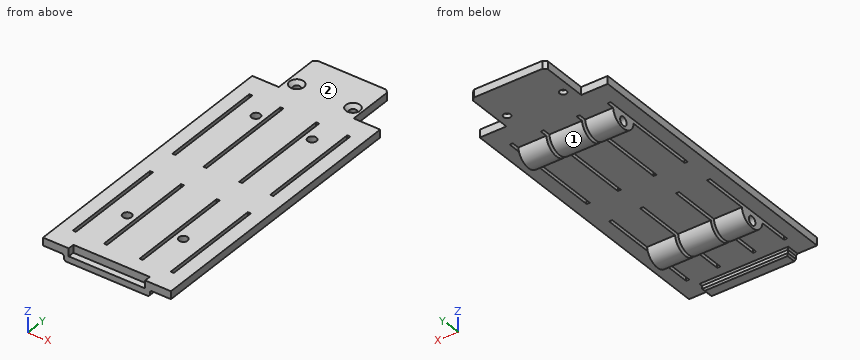
```python
from build123d import *

# Parameters (mm, degrees)
BOSS_EXTRU_1_DEPTH              = 2.5
BOSS_EXTRU_2_DEPTH              = 30.59
ESQUISSE5_W                     = 2
ESQUISSE5_H                     = 67
ENL_V_MAT_EXTRU_1_DEPTH         = 130.359962894
ESQUISSE14_W                    = 49
ESQUISSE14_H                    = 4
ENL_V_MAT_EXTRU_5_DEPTH         = 129.953479984
R_P_TITION_LIN_AIRE2_COUNT      = 2
R_P_TITION_LIN_AIRE2_PITCH      = 19.921
ESQUISSE17_R                    = 2.25
ENL_V_MAT_EXTRU_7_DEPTH         = 10
ESQUISSE15_W                    = 55
ESQUISSE15_H                    = 7
BOSS_EXTRU_4_DEPTH              = 4
CHANFREIN3_SIZE                 = 1
CHANFREIN4_SIZE                 = 2
ESQUISSE19_R                    = 2.8
ENL_V_MAT_EXTRU_9_DEPTH         = 8
CHANFREIN5_SIZE                 = 2.3
SYM_TRIE9_COPY_1_SKETCH_W       = 2
SYM_TRIE9_COPY_1_SKETCH_H       = 67
SYM_TRIE9_COPY_1_DEPTH          = 130.359962894
ESQUISSE20_R                    = 2.8
ENL_V_MAT_EXTRU_10_DEPTH        = 10
R_P_TITION_LIN_AIRE3_COUNT      = 2
R_P_TITION_LIN_AIRE3_PITCH      = 36
R_P_TITION_LIN_AIRE3_COUNT_DIR2 = 2
R_P_TITION_LIN_AIRE3_PITCH_DIR2 = 112


with BuildPart() as part:
    # Esquisse1 → Boss.-Extru.1 (new, symmetric)
    with BuildSketch(Plane.XY):
        Polygon((-41, -91), (-15.008, -91), (41, -91), (41, 91), (24, 91), (24, 122), (-24, 122), (-24, 91), (-41, 91), align=None)
    extrude(amount=BOSS_EXTRU_1_DEPTH, both=True)

    # Esquisse6 → Boss.-Extru.2 (add, symmetric)
    with BuildSketch(Plane(origin=(0, 0, 0), x_dir=(0, 0, -1), z_dir=(1, 0, 0))):
        with BuildLine():
            Line((2.5, -57.94427191), (2.5, -40.05572809))
            ThreePointArc((2.5, -40.05572809), (10.5, -49), (2.5, -57.94427191))
        make_face()
        with BuildLine():
            Line((2.5, 54.05572809), (2.5, 71.94427191))
            ThreePointArc((2.5, 71.94427191), (10.5, 63), (2.5, 54.05572809))
        make_face()
    extrude(amount=BOSS_EXTRU_2_DEPTH, both=True)

    # Esquisse5 → Enlèv. mat.-Extru.1 (cut, symmetric)
    with BuildSketch(Plane.XY.offset(2.5)):
        with Locations((31.3815, -43.25)):
            Rectangle(ESQUISSE5_W, ESQUISSE5_H)
        with Locations((31.3815, 43.25)):
            Rectangle(ESQUISSE5_W, ESQUISSE5_H)
    enl_v_mat_extru_1 = extrude(amount=ENL_V_MAT_EXTRU_1_DEPTH, both=True, mode=Mode.SUBTRACT)

    # Esquisse14 → Enlèv. mat.-Extru.5 (cut, through all)
    with BuildSketch(Plane(origin=(0, 0, -2.5), x_dir=(-1, 0, 0), z_dir=(0, 0, -1))):
        with Locations((0, -89)):
            Rectangle(ESQUISSE14_W, ESQUISSE14_H)
    extrude(amount=-ENL_V_MAT_EXTRU_5_DEPTH, mode=Mode.SUBTRACT)

    # Répétition linéaire2: Enlèv. mat.-Extru.1 ×2
    with Locations(*[(-i * R_P_TITION_LIN_AIRE2_PITCH, 0, 0) for i in range(1, R_P_TITION_LIN_AIRE2_COUNT)]):
        add(enl_v_mat_extru_1, mode=Mode.SUBTRACT)

    # Esquisse17 → Enlèv. mat.-Extru.7 (cut)
    with BuildSketch(Plane.XY.offset(2.5)):
        with Locations((18, 98.55)):
            Circle(ESQUISSE17_R)
        with Locations((-18, 98.55)):
            Circle(ESQUISSE17_R)
    extrude(amount=-ENL_V_MAT_EXTRU_7_DEPTH, mode=Mode.SUBTRACT)

    # Esquisse15 → Boss.-Extru.4 (add)
    with BuildSketch(Plane(origin=(0, 0, -2.5), x_dir=(-1, 0, 0), z_dir=(0, 0, -1))):
        with Locations((0, -87.5)):
            Rectangle(ESQUISSE15_W, ESQUISSE15_H)
    extrude(amount=BOSS_EXTRU_4_DEPTH)

    # Chanfrein3
    chanfrein3_edges = [part.edges().sort_by_distance(p)[0] for p in [
        (27.5, -87.5, -2.5),
        (-27.5, -87.5, -2.5),
        (0, -84, -2.5),
        (27.5, -87.5, -6.5),
        (-27.5, -87.5, -6.5),
        (0, -84, -6.5),
    ]]
    chamfer(chanfrein3_edges, length=CHANFREIN3_SIZE)

    # Chanfrein4
    chanfrein4_edges = [part.edges().sort_by_distance(p)[0] for p in [
        (-24, 122, 0),
        (24, 122, 0),
    ]]
    chamfer(chanfrein4_edges, length=CHANFREIN4_SIZE)

    # Esquisse19 → Enlèv. mat.-Extru.9 (cut)
    with BuildSketch(Plane(origin=(30.3815, 0, 0), x_dir=(0, 0, -1), z_dir=(1, 0, 0))):
        with Locations(Location((6, 63, 0), (0, 0, 90))):
            Circle(ESQUISSE19_R)
        with Locations(Location((6, -49, 0), (0, 0, 90))):
            Circle(ESQUISSE19_R)
    enl_v_mat_extru_9 = extrude(amount=-ENL_V_MAT_EXTRU_9_DEPTH, mode=Mode.SUBTRACT)

    # Symétrie8: Enlèv. mat.-Extru.9 across plane
    add(enl_v_mat_extru_9.mirror(Plane(origin=(0, 0, 0), x_dir=(0, 0, 1), z_dir=(1, 0, 0))), mode=Mode.SUBTRACT)

    # Chanfrein5
    chanfrein5_edges = [part.edges().sort_by_distance(p)[0] for p in [
        (15.75, 98.55, 2.5),
        (-20.25, 98.55, 2.5),
    ]]
    chamfer(chanfrein5_edges, length=CHANFREIN5_SIZE)

    # Symétrie9: Enlèv. mat.-Extru.1 across plane
    add(enl_v_mat_extru_1.mirror(Plane(origin=(0, 0, 0), x_dir=(0, 0, 1), z_dir=(1, 0, 0))), mode=Mode.SUBTRACT)

    # Symétrie9 copy 1 sketch → Symétrie9 copy 1 (cut, symmetric)
    with BuildSketch(Plane(origin=(19.921, 0, 2.5), x_dir=(-1, 0, 0), z_dir=(0, 0, 1))):
        with Locations((31.3815, 43.25)):
            Rectangle(SYM_TRIE9_COPY_1_SKETCH_W, SYM_TRIE9_COPY_1_SKETCH_H)
        with Locations((31.3815, -43.25)):
            Rectangle(SYM_TRIE9_COPY_1_SKETCH_W, SYM_TRIE9_COPY_1_SKETCH_H)
    extrude(amount=SYM_TRIE9_COPY_1_DEPTH, both=True, mode=Mode.SUBTRACT)

    # Esquisse20 → Enlèv. mat.-Extru.10 (cut)
    with BuildSketch(Plane.XY.offset(2.5)):
        with Locations((-18, -49)):
            Circle(ESQUISSE20_R)
    enl_v_mat_extru_10 = extrude(amount=-ENL_V_MAT_EXTRU_10_DEPTH, mode=Mode.SUBTRACT)

    # Répétition linéaire3: Enl_v. mat.-Extru.10 2 × 2
    with Locations(*[(i * R_P_TITION_LIN_AIRE3_PITCH, j * R_P_TITION_LIN_AIRE3_PITCH_DIR2, 0) for i in range(R_P_TITION_LIN_AIRE3_COUNT) for j in range(R_P_TITION_LIN_AIRE3_COUNT_DIR2) if (i, j) != (0, 0)]):
        add(enl_v_mat_extru_10, mode=Mode.SUBTRACT)


solid = part.part
```
Source: CAD feature listing. Evaluate the final solid. Frame: model axes, mm. Face numbers are marked on the shaded views. Give positions to 0.01 mm unless a question says otherwise; leave off trailing zeros. Order: outer loops, then holes, each group sorted by start corner. A loop starts at its lowest first (then second) coordinate and runs counter-clockwise, first axis right, second up.
(1) Section query C-C (x = 1). Return the cut outline in (y, z).
(2) Contact query for flat-ended pins moving along their axis: P1, Ø3.5, axis at x = 18, y = 63, coming from the +Z side; P2, Ø5.5, axis at y = 110, z = 0, coming from the +X side; P3, Ø2, axis at y = -45, z = -5.5, coming from the -X side; P4, Ø6.5, axis at y = 44, z = -6.5, coming from the +X side. Output: stop coordinate, or through.
(3) Section query B-B (y = 98.55). Return the cut outline in (x, z).
(4) Material intervals for line 1 along Y through (x, z) = (-18, -1.4); line 2 along X through (y, z) = (72, -1.5); line 3 along Y through (x, z) = (-18, -5.5), sorted ascending.
(5) Section query D-D (y = 63). State how many separate pieces and enclosed holes the cut face has, plus the area to 3 significant figures.
(6) Pull-direction query (Y, two-part tool) for the marked faces 1 and 2; classes: +Y half, -Y half, draft (parallel to the pull), parting line (faces both ways), or undercut.
(7) Section query A-A (x = 18). Return the cut outline in (y, z).
Outcome:
1. outline: (-91, -6.5) - (-85, -6.5) - (-84, -5.5) - (-84, -3.5) - (-83, -2.5) - (-57.94, -2.5) arc R9 ccw to (-40.06, -2.5) - (54.06, -2.5) arc R9 ccw to (71.94, -2.5) - (122, -2.5) - (122, 2.5) - (-87, 2.5) - (-87, -2.5) - (-91, -2.5) - close
2. P1: stops at z = -7.5
2. P2: stops at x = 24
2. P3: stops at x = -30.38
2. P4: passes through
3. outline: (-24, -2.5) - (-20.25, -2.5) - (-20.25, 0.2) - (-22.55, 2.5) - (-24, 2.5) - close; (-15.75, -2.5) - (15.75, -2.5) - (15.75, 0.2) - (13.45, 2.5) - (-13.45, 2.5) - (-15.75, 0.2) - close; (20.25, -2.5) - (24, -2.5) - (24, 2.5) - (22.55, 2.5) - (20.25, 0.2) - close
4. line 1: y = -87 to -51.8, -46.2 to 60.2, 65.8 to 96.3, 100.8 to 122
4. line 2: x = -41 to -32.38, -30.38 to -12.46, -10.46 to 10.46, 12.46 to 30.38, 32.38 to 41
4. line 3: y = -91 to -84, -57.06 to -51.8, -46.2 to -40.94, 54.94 to 60.2, 65.8 to 71.06
5. separate pieces: 5
5. enclosed holes: 0
5. area: 623 mm2
6. face 1: undercut
6. face 2: draft
7. outline: (-91, -6.5) - (-85, -6.5) - (-84, -5.5) - (-84, -3.5) - (-83, -2.5) - (-57.94, -2.5) arc R9 ccw to (-40.06, -2.5) - (54.06, -2.5) arc R9 ccw to (71.94, -2.5) - (96.3, -2.5) - (96.3, 0.2) - (94, 2.5) - (65.8, 2.5) - (65.8, -7.5) - (60.2, -7.5) - (60.2, 2.5) - (-46.2, 2.5) - (-46.2, -7.5) - (-51.8, -7.5) - (-51.8, 2.5) - (-87, 2.5) - (-87, -2.5) - (-91, -2.5) - close; (100.8, -2.5) - (122, -2.5) - (122, 2.5) - (103.1, 2.5) - (100.8, 0.2) - close
